from build123d import *

# Parameters (mm, degrees)
SKETCH_1_R          = 4.15
EXTRUDE_1_DEPTH     = 3
EXTRUDE_2_DEPTH     = 12
CUT_EXTRUDE_1_DEPTH = 112.858735101
CUT_EXTRUDE_2_DEPTH = 112.858735101


with BuildPart() as part:
    # 草图1 → 凸台-拉伸1 (new body)
    with BuildSketch(Plane(origin=(0, 0, 0), x_dir=(1, 0, 0), z_dir=(0, 1, 0))):
        with BuildLine():
            ThreePointArc((19.532394726, 15.60402372), (-17.67766953, 17.67766953), (-15.60402372, -19.532394726))
            Line((-15.60402372, -19.532394726), (54.277196075, -75.359047143))
            ThreePointArc((54.277196075, -75.359047143), (74.246212025, -74.246212025), (75.359047143, -54.277196075))
            Line((75.359047143, -54.277196075), (19.532394726, 15.60402372))
        make_face()
        with Locations(Location((0, 0, 0), (0, 0, 270))):
            Circle(SKETCH_1_R, mode=Mode.SUBTRACT)
        with Locations(Location((63.639610307, -63.639610307, 0), (0, 0, 270))):
            Circle(SKETCH_1_R, mode=Mode.SUBTRACT)
    extrude(amount=EXTRUDE_1_DEPTH)

    # 草图3 → 凸台-拉伸2 (add)
    with BuildSketch(Plane(origin=(0, 3, 0), x_dir=(1, 0, 0), z_dir=(0, 1, 0))):
        with BuildLine():
            ThreePointArc((54.277196075, -75.359047143), (74.246212025, -74.246212025), (75.359047143, -54.277196075))
            Line((75.359047143, -54.277196075), (19.532394726, 15.60402372))
            ThreePointArc((19.532394726, 15.60402372), (-17.67766953, 17.67766953), (-15.60402372, -19.532394726))
            Line((-15.60402372, -19.532394726), (54.277196075, -75.359047143))
        make_face()
        with BuildLine():
            Line((17.969803148, 14.355701822), (73.796455565, -55.525517972))
            ThreePointArc((73.796455565, -55.525517972), (72.831998462, -72.831998462), (55.525517972, -73.796455565))
            Line((55.525517972, -73.796455565), (-14.355701822, -17.969803148))
            ThreePointArc((-14.355701822, -17.969803148), (-16.263455967, 16.263455967), (17.969803148, 14.355701822))
        make_face(mode=Mode.SUBTRACT)
    extrude(amount=EXTRUDE_2_DEPTH)

    # 草图4 → 切除-拉伸1 (cut, through all)
    with BuildSketch(Plane(origin=(0, 3, 0), x_dir=(1, 0, 0), z_dir=(0, 1, 0))):
        Polygon((17.133662373, -2.976992155), (10.055327264, -10.055327264), (54.909619217, -54.909619217), (61.987954325, -47.831284108), align=None)
        Polygon((54.909619217, -54.909619217), (10.055327264, -10.055327264), (2.529939412, -17.580715117), (47.384231364, -62.435007069), align=None)
    extrude(amount=-CUT_EXTRUDE_1_DEPTH, mode=Mode.SUBTRACT)

    # 草图5 → 切除-拉伸2 (cut, through all)
    with BuildSketch(Plane(origin=(0, 3, 0), x_dir=(1, 0, 0), z_dir=(0, 1, 0))):
        with BuildLine():
            Line((-6.700597737, -24.085306516), (-14.355701822, -17.969803148))
            ThreePointArc((-14.355701822, -17.969803148), (-16.263455967, 16.263455967), (17.969803148, 14.355701822))
            Line((17.969803148, 14.355701822), (24.085306516, 6.700597737))
            ThreePointArc((24.085306516, 6.700597737), (22.258564958, 11.382279474), (19.532394726, 15.60402372))
            ThreePointArc((19.532394726, 15.60402372), (-17.67766953, 17.67766953), (-15.60402372, -19.532394726))
            ThreePointArc((-15.60402372, -19.532394726), (-11.382279474, -22.258564958), (-6.700597737, -24.085306516))
        make_face()
        with BuildLine():
            Line((24.085306516, 6.700597737), (69.125662715, -49.678835652))
            ThreePointArc((69.125662715, -49.678835652), (72.544296976, -51.568713268), (75.359047143, -54.277196075))
            Line((75.359047143, -54.277196075), (19.532394726, 15.60402372))
            ThreePointArc((19.532394726, 15.60402372), (22.258564958, 11.382279474), (24.085306516, 6.700597737))
        make_face()
        with BuildLine():
            Line((49.678835652, -69.125662715), (-6.700597737, -24.085306516))
            ThreePointArc((-6.700597737, -24.085306516), (-11.382279474, -22.258564958), (-15.60402372, -19.532394726))
            Line((-15.60402372, -19.532394726), (54.277196075, -75.359047143))
            ThreePointArc((54.277196075, -75.359047143), (51.568713268, -72.544296976), (49.678835652, -69.125662715))
        make_face()
        with BuildLine():
            ThreePointArc((75.359047143, -54.277196075), (72.544296976, -51.568713268), (69.125662715, -49.678835652))
            Line((69.125662715, -49.678835652), (73.796455565, -55.525517972))
            ThreePointArc((73.796455565, -55.525517972), (75.908248951, -59.340714422), (76.639610307, -63.639610307))
            ThreePointArc((76.639610307, -63.639610307), (69.275069456, -75.354626319), (55.525517972, -73.796455565))
            Line((55.525517972, -73.796455565), (49.678835652, -69.125662715))
            ThreePointArc((49.678835652, -69.125662715), (51.568713268, -72.544296976), (54.277196075, -75.359047143))
            ThreePointArc((54.277196075, -75.359047143), (70.142063172, -77.156936475), (78.639610307, -63.639610307))
            ThreePointArc((78.639610307, -63.639610307), (77.795731819, -58.679345825), (75.359047143, -54.277196075))
        make_face()
    extrude(amount=CUT_EXTRUDE_2_DEPTH, mode=Mode.SUBTRACT)


solid = part.part
Could you check a few things on this model? Use its own coordinates, in mm. A direction names the side the tool comes from. Give positions to 0.01 mm unless a question says otherwise; leave off trailing zeros. Write each loop counter-clockwise with the first axis right and the second up, starting at its lowest first coordinate (ties: lowest second). Pieces come first, ordered by that corner, then holes. Notation, with made-up numbers: (9.5, 73) -> (40.5, 73) arc R28 ccw to (40.5, 95) -> close; hole circle Ø7 at (61, -14.75). An arc over 180 degrees is marked (long way). Write each question's results on one line, items separated by ' | '. Start each with the question number.
Q1. Suppose I cut it at B-B, the plane z = 14. List the corners of the cut face in (x, y) for me.
Q2. I need wall thicknesses on probe 1 along X at (y, z) = (1.15, 32); probe 2 along Z at (x, y) = (20, 1.1); probe 3 along X at (y, z) = (2.8, 25.5). Which ranges of each line are inside material? Lowest first, please.
Q3. Suppose I cut it at D-D, the plane x = -11.5. List the corners of the cut face in (y, z) for me, and give its area (3 significant figures).
Q4. We'd pull the mould along X, two halves only. Please class faces 3 (the face through (74.03, 1.48, 74.46)), 4 (the face through (30, 0, 15)), 5 (the face through (39.875, 1.521, 25.718)): +X half, -X half, draft (parallel to the pull), parting line (faces both ways), or undercut.
Q5. I'm going to push a flat-ended pin straight in: pin 1 Ø1.5 at (x, y) = (40, 2) entering from +Z. Where does the tip first touch, or does it pass through?
Q6. Suppose I cut it at C-C, the plane y = 1.2. List the corners of the cut face in (x, z) for me (3 decimals), and give its area (3 significant figures).
Q7. Suppose I cut it at A-A, the plane x = 25.5. List the corners of the cut face in (y, z) for me, and give its area (3 significant figures).
Q8. Which directions (+Z, -Z, +X, -X, +Y, -Y) give clear straight access to the entire face, cutting with the end or side of a thin tool? Please do faces 1 (the face through (18.847, 1.479, 47.055)), 2 (the face through (24.64, 1.52, 39.69)).
Outcome:
1) outline: (-20.71, 0) -> (6.11, 0) -> (6.11, 3) -> (-20.71, 3) -> close; (28.16, 0) -> (43.18, 0) -> (43.18, 3) -> (28.16, 3) -> close
2) probe 1: 0 to 16.95, 46.16 to 57.56 | probe 2: -15.02 to 5.84, 35.05 to 47.98 | probe 3: -8.13 to 10.45, 39.66 to 52.37
3) outline: (0, -22.2) -> (3, -22.2) -> (3, 22.81) -> (0, 22.81) -> close | area: 135 mm2
4) face 3: parting line | face 4: draft | face 5: undercut
5) pin 1: z = 64.55
6) outline: (-15.604, 19.532) arc R25 ccw (long way) to (19.532, -15.604) -> (75.359, 54.277) arc R15 ccw to (54.277, 75.359) -> close; hole circle Ø8.3 at (0, 0); hole (2.53, 17.581) -> (17.134, 2.977) -> (61.988, 47.831) -> (47.384, 62.435) -> close; hole circle Ø8.3 at (63.64, 63.64) | area: 3,540 mm2
7) outline: (0, -8.13) -> (3, -8.13) -> (3, 11.34) -> (0, 11.34) -> close; (0, 40.55) -> (3, 40.55) -> (3, 52.37) -> (0, 52.37) -> close | area: 93.9 mm2
8) face 1: +Z, -X, +Y, -Y | face 2: +Y, -Y
